Design review of the part shown in the three views and the two pictorial views. Dimensions are in mm from the part's minimum x, y and z. A direction names the side the tool comes from. Give positions to 0.01 mm unless a question says otherwise; leave off trailing zeros. Write each loop counter-clockwise with the first axis right and the second up, starting at its lowest first coordinate (ties: lowest second). Pieces come first, ordered by that corner, then holes.
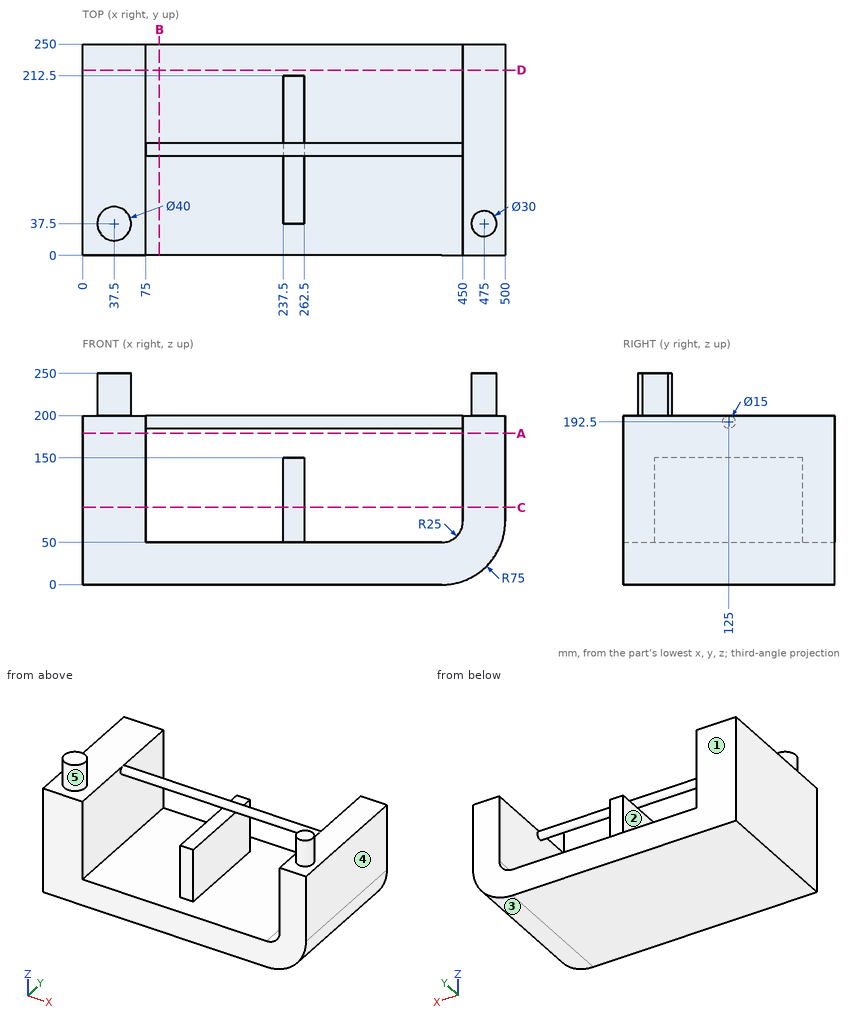
(1) Mouldability with a two-part tool opening along X and no side actions: class the marked faces 1, 2 and 3 as pulls with the +X half, pulls with the -X half, needs draft (parallel to the pull), parting line crosses it, or undercut.
Resolved:
face 1: needs draft
face 2: undercut
face 3: pulls with the +X half
(2) Consider section A-A, the plane z = 179. Give the boundary of the cut face in (x, y), then the cut area to 4 significant figures.
Resolved:
outline: (0, 0) - (75, 0) - (75, 250) - (0, 250) - close; (450, 0) - (500, 0) - (500, 250) - (450, 250) - close
area: 31,250 mm2
(3) Tool access review of the marked faces 4 and 5: name each direction out of +Z, -Z, +X, -X, +Y, -Y from which nothing blocks a thin tool from reaching the whole face with its end or side.
Resolved:
face 4: +Z, -Z, +X, +Y, -Y
face 5: +Z
(4) Consider section B-B, the plane x = 91. Give the boundary of the cut face in (y, z).
Resolved:
outline: (0, 0) - (250, 0) - (250, 50) - (0, 50) - close; circle Ø15 at (125, 192.5)
(5) Consider section C-C, the plane z = 91.5. Give the boundary of the cut face in (x, y), then the cut area to 3 significant figures.
Resolved:
outline: (0, 0) - (75, 0) - (75, 250) - (0, 250) - close; (237.5, 37.5) - (262.5, 37.5) - (262.5, 212.5) - (237.5, 212.5) - close; (450, 0) - (500, 0) - (500, 250) - (450, 250) - close
area: 35,600 mm2
(6) Consider section D-D, the plane y = 219. Give the boundary of the cut face in (x, z).
Resolved:
outline: (0, 0) - (425, 0) arc R75 ccw to (500, 75) - (500, 200) - (450, 200) - (450, 75) arc R25 cw to (425, 50) - (75, 50) - (75, 200) - (0, 200) - close
(7) To check wall thickness, follow L1, parallel to X at y = 124, z = 125; L2, parallel to X at y = 173, z = 169; L3, parallel to X at y = 184, z = 54. State the ranges of each line that lie inside material, in increasing order.
Resolved:
L1: x = 0 to 75, 237.5 to 262.5, 450 to 500
L2: x = 0 to 75, 450 to 500
L3: x = 0 to 75, 237.5 to 262.5, 438.56 to 497
(8) Clearance check with flat-ended pins moving along their axes: P1, Ø6, axis at y = 120, z = 32, coming from the -X side; P2, Ø22.5, axis at x = 55, y = 104, coming from the +Z side; P3, Ø12.5, axis at x = 252, z = 109, coming from the +Y side. State where each tip first meets the part, or that it passes through.
Resolved:
P1: stops at x = 0
P2: stops at z = 200
P3: stops at y = 212.5
